from build123d import *

# Parameters (mm, degrees)
SKETCH_4_R                = 40
CUT_EXTRUDE_1_DEPTH       = 407.201920232
HOLE_WIZARD_1_D           = 3.4
HOLE_WIZARD_1_DEPTH       = 8
HOLE_WIZARD_1_CBORE_D     = 6
HOLE_WIZARD_1_CBORE_DEPTH = 3.4
PATTERN_CIRCULAR_1_COUNT  = 12
HOLE_WIZARD_3_D           = 3.4
HOLE_WIZARD_3_DEPTH       = 8
HOLE_WIZARD_3_CBORE_D     = 6
HOLE_WIZARD_3_CBORE_DEPTH = 3.4
PATTERN_CIRCULAR_2_COUNT  = 12
CHAMFER_1_SIZE            = 0.5


with BuildPart() as part:
    # 草图3 → 旋转1 (revolve)
    with BuildSketch(Plane.XY, mode=Mode.PRIVATE) as revolve_1_sk:
        Polygon((0, 0), (0, 50), (8, 50), (8, 42.5), (392, 42.5), (392, 50), (400, 50), (400, 0), align=None)
    revolve(revolve_1_sk.sketch.rotate(Axis((-303.553299492, 0, 0), (1, 0, 0)), 90), axis=Axis((-303.553299492, 0, 0), (1, 0, 0)))

    # 草图4 → 切除-拉伸1 (cut, through all)
    with BuildSketch(Plane(origin=(400, 0, 0), x_dir=(0, 0, -1), z_dir=(1, 0, 0))):
        Circle(SKETCH_4_R)
    extrude(amount=-CUT_EXTRUDE_1_DEPTH, mode=Mode.SUBTRACT)

    # 打孔尺寸(%根据)内六角圆柱头螺钉的类型1
    with Locations(Plane.ZY.offset(-392)):
        with Locations((0, 46)):
            hole_wizard_1 = CounterBoreHole(HOLE_WIZARD_1_D / 2, HOLE_WIZARD_1_CBORE_D / 2, HOLE_WIZARD_1_CBORE_DEPTH, depth=HOLE_WIZARD_1_DEPTH)

    # 阵列(圆周)1: 打孔尺寸(%根据)内六角圆柱头螺钉的类型1 ×12 about axis
    pattern_circular_1_axis = Axis((0, 0, 0), (1, 0, 0))
    for i in range(1, PATTERN_CIRCULAR_1_COUNT):
        add(hole_wizard_1.rotate(pattern_circular_1_axis, i * 360 / PATTERN_CIRCULAR_1_COUNT), mode=Mode.SUBTRACT)

    # 打孔尺寸(%根据)内六角圆柱头螺钉的类型3
    with Locations(Plane(origin=(8, 0, 0), x_dir=(0, 0, -1), z_dir=(1, 0, 0))):
        with Locations((0, 46)):
            hole_wizard_3 = CounterBoreHole(HOLE_WIZARD_3_D / 2, HOLE_WIZARD_3_CBORE_D / 2, HOLE_WIZARD_3_CBORE_DEPTH, depth=HOLE_WIZARD_3_DEPTH)

    # 阵列(圆周)2: 打孔尺寸(%根据)内六角圆柱头螺钉的类型3 ×12 about axis
    pattern_circular_2_axis = Axis((0, 0, 0), (1, 0, 0))
    for i in range(1, PATTERN_CIRCULAR_2_COUNT):
        add(hole_wizard_3.rotate(pattern_circular_2_axis, i * 360 / PATTERN_CIRCULAR_2_COUNT), mode=Mode.SUBTRACT)

    # 倒角1
    chamfer_1_edges = [part.edges().sort_by_distance(p)[0] for p in [
        (392, 0, -50),
        (8, 0, -50),
    ]]
    chamfer(chamfer_1_edges, length=CHAMFER_1_SIZE)


solid = part.part
Geometry: final body of the model. Coordinates: model frame, mm. A direction names the side the tool comes from. Give positions to 0.01 mm unless a question says otherwise; leave off trailing zeros. Write each loop counter-clockwise with the first axis right and the second up, starting at its lowest first coordinate (ties: lowest second). Pieces come first, ordered by that corner, then holes. Notation, with made-up numbers: M 73.25,-15.75 L 101.25,-15.75 A38 cw 101.25,22.25 Z; hole C 4.5,65.25 d7. An arc over 180 degrees is marked long. Answer in a Markdown table with one row per item. Add a question column.
(1) First-contact query: pin 1 (12 mm diameter, centred on x = 146.5, z = -2.5, fed in from -Y); pin 2 (5 mm diameter, centred on x = 327.5, z = 24, fed in from -Y); pin 3 (4 mm diameter, centred on x = 214, z = 6, fed in from -Y). Flat tips, straight axial feed; report the tip coordinate or a pass-through.
(2) Mould query, pull axis X, two halves, no side actions, for faces 1 (the flat face through (400, -15, -37.3)), 2 (the flat face through (0, -15, 37.3)), 3 (the flat face through (8, 40, -15)). Classes: +X half, -X half, draft (parallel to the pull), parting line (faces both ways), or undercut.
(3) Section A-A on x = 366.5. Return loops of the section in (y, z).
(4) Reachability of faces 4 (the cylindrical face through (202.688, -12.766, 40.537)), 5 (the cylindrical face through (202.8, -39.05, 8.67)) from +Z, -Z, +X, -X, +Y, -Y: full face, straight path, thin tool, end or side. Return the list, or none.
(5) Ray query, line 1 (X direction, y = -33.5, z = 36); line 2 (Y direction, x = 394, z = -23); line 3 (Z direction, x = 273, y = -3.5). Return the intervals inside material, ascending.
Result set:
| question | item | result |
|---|---|---|
| 1 | pin 1 | stops at y = -42.5 |
| 1 | pin 2 | stops at y = -36.66 |
| 1 | pin 3 | stops at y = -42.31 |
| 2 | face 1 | +X half |
| 2 | face 2 | -X half |
| 2 | face 3 | undercut |
| 3 | outline | C 0,0 d85; hole C 0,0 d80 |
| 4 | face 4 | none |
| 4 | face 5 | +X, -X |
| 5 | line 1 | x = 0 to 8, 392 to 400 |
| 5 | line 2 | y = -44.4 to -42.84, -36.84 to -32.73, 32.73 to 36.84, 42.84 to 44.4 |
| 5 | line 3 | z = -42.36 to -39.85, 39.85 to 42.36 |
